Part model, mm, in its own coordinate system. A direction names the side the tool comes from. Round coordinates to 2 decimals unless told otherwise and drop trailing zeros. Write each loop counter-clockwise with the first axis right and the second up, starting at its lowest first coordinate (ties: lowest second). Pieces come first, ordered by that corner, then holes. Notation, with made-up numbers: (85, -39.75) -> (96, -39.75) arc R6 ccw to (96, -35.75) -> close; hole circle Ø6 at (20, -23). An arc over 180 degrees is marked (long way). Use CSV: the item, a comma, the result in double quotes. Start each with the question number.
(1) Two-plate mould, pull along Z, no slides. Class faces 6 (the flat face through (61, 3, -84)), 7 (the flat face through (61, 10, -65)), 8 (the flat face through (60, 9, -55)), 9 (the cylindrical face through (62.9, 1.5, -73.2)): released by +Z, released by -Z, zero draft, split by the parting line, or undercut.
(2) Which spindle directions (+Z, -Z, +X, -X, +Y, -Y) get a long thin tool onto all of the face, cutting with end or side? Do faces 1 (the flat face through (93.5, 10, -40)), 2 (the flat face through (27.5, 10, -40)), 3 (the flat face through (33, 12, -15)), 4 (the flat face through (78.5, 16, -35)), 5 (the flat face through (37.4, 7.9, -34.7)). Say none if no direction does.
(3) Saw through at B-B (z = -75). Give the cut face in (x, y), plus the area to 3 significant figures.
(4) Drop flat-ended pins along their axis: pin 1 (9.5 mm diameter, centred on x = 60.5, z = -75, fed in from +Y); pin 2 (4.5 mm diameter, centred on y = 10.5, z = -34, fed in from +X); pin 3 (4 mm diameter, centred on x = 52.5, y = 15, fed in from -Z). Give the stop position or say it passes through.
(5) Saw through at A-A (x = 60.5). Give the cut face in (y, z).
(6) Saw through at C-C (y = 5). Give the cut face in (x, z).
(7) Probe line 1 (Z direction, x = 60.5, y = 1.8); line 2 (Z direction, x = 55, y = 4.5); line 3 (Y direction, x = 61.5, z = -130.5). List the from-to ranges inside material, lowest first. Write a range as [from, to].
(8) Saw through at D-D (x = 30.5). Give the cut face in (y, z).
Autodesk Inventor part; units mm, degrees
ref_plane "YZ Plane" through (0, 0, 0) normal (1, 0, 0) x (0, 1, 0)
ref_plane "XZ Plane" through (0, 0, 0) normal (0, 1, 0) x (-1, 0, 0)
ref_plane "XY Plane" through (0, 0, 0) normal (0, 0, 1) x (1, 0, 0)
sketch "Skizze1" plane through (0, 0, 0) normal (0, 1, 0) x (-1, 0, 0)
  line L0 (0, 0) -> (-121, 0)
  line L1 (-121, 0) -> (-121, -170)
  line L2 (-121, -170) -> (0, -170)
  line L3 (0, -170) -> (0, 0)
  circle A0 centre (-60.5, -75) radius 3
  circle A1 centre (-60.5, -124.75) radius 2.75
  dimension "d0" = 121
  dimension "d1" = 170
  dimension "d2" = 75
  dimension "d3" = 6
  dimension "d4" = 60.5
  dimension "d5" = 49.75
  dimension "d6" = 60.5
  dimension "d7" = 5.5
extrude "Extrusion1" add sketch "Skizze1" along normal blind 3
sketch "Skizze6" plane through (0, 3, 0) normal (0, 1, 0) x (1, 0, 0)
  line L0 (27.5, 15) -> (93.5, 15)
  line L1 (93.5, 15) -> (93.5, 65)
  line L2 (93.5, 65) -> (27.5, 65)
  line L3 (27.5, 65) -> (27.5, 15)
  line L4 (0, 170) -> (0, 0)
  line L5 (0, 0) -> (121, 0)
  dimension "d72" = 66
  dimension "d73" = 50
  dimension "d74" = 27.5
  dimension "d75" = 15
extrude "Extrusion6" add sketch "Skizze6" along normal blind 15
sketch "Skizze7" plane through (27.5, 3, -15) normal (0, 0, 1) x (1, 0, 0)
  line L0 (66, 15) -> (0, 15)
  line L1 (0, 0) -> (66, 0)
  line L2 (15, 15) -> (51, 15)
  line L3 (51, 15) -> (51, 0)
  line L4 (51, 0) -> (15, 0)
  line L5 (15, 0) -> (15, 15)
  line L6 (0, 0) -> (0, 15)
  line L7 (0, 0) -> (21.2132, 0) construction
  line L8 (66, 0) -> (87.2132, 0) construction
  line L9 (66, 0) -> (66, 15)
  line L10 (93.5, 0) -> (-27.5, 0)
  line L11 (5, 0) -> (15, 10)
  line L12 (5, 0) -> (19.1421, 0) construction
  line L13 (51, 10) -> (61, 0)
  line L14 (51, 10) -> (65.1421, 10) construction
  line L15 (15, 15) -> (51, 15)
  line L16 (51, 15) -> (51, 10)
  line L17 (51, 10) -> (15, 10)
  line L18 (15, 10) -> (15, 15)
  point P0 (-27.5, -3)
  dimension "d78" = 36
  dimension "d79" = 15
  dimension "d85" = 45
  dimension "d86" = 45
extrude "Extrusion7" cut sketch "Skizze7" against normal blind 40 contours L3 L17 L5 L0 | L13 L1 L3 | L3 L1 L5 L17 | L5 L1 L11
sketch "Skizze8" plane through (0, 3, 0) normal (0, 1, 0) x (1, 0, 0)
  point P0 (0, 0)
properties part number "platform-mount"
Answers:
1,face 6,"zero draft"
1,face 7,"released by -Z"
1,face 8,"released by +Z"
1,face 9,"undercut"
2,face 1,"+Z, -Z, +X, +Y"
2,face 2,"+Z, -Z, -X, +Y"
2,face 3,"+Z, +X, -X, +Y"
2,face 4,"+Z, +Y"
2,face 5,"+Z"
3,outline,"(0, 0) -> (57.5, 0) -> (57.5, 3) -> (0, 3) -> close; (63.5, 0) -> (121, 0) -> (121, 3) -> (63.5, 3) -> close"
3,area,"345 mm²"
4,pin 1,"stops at y = 3"
4,pin 2,"stops at x = 93.5"
4,pin 3,"stops at z = -65"
5,outline,"(0, -170) -> (3, -170) -> (3, -127.5) -> (0, -127.5) -> close; (0, -122) -> (3, -122) -> (3, -78) -> (0, -78) -> close; (0, -72) -> (3, -72) -> (3, -65) -> (18, -65) -> (18, -55) -> (3, -55) -> (3, 0) -> (0, 0) -> close"
6,outline,"(27.5, -65) -> (93.5, -65) -> (93.5, -15) -> (86.5, -15) -> (86.5, -55) -> (34.5, -55) -> (34.5, -15) -> (27.5, -15) -> close"
7,line 1,"z = [-170, -127.5], [-122, -78], [-72, 0]"
7,line 2,"z = [-65, -55]"
7,line 3,"y = [0, 3]"
8,outline,"(0, -170) -> (3, -170) -> (3, -65) -> (18, -65) -> (18, -15) -> (3, -15) -> (3, 0) -> (0, 0) -> close"
